The figure shows three views and two pictorial views of one solid part (mm, origin at its lowest corner). Answer the questions. Coordinates: 2 decimals unless noted, no trailing zeros. Order: outer loops, then holes, each group sorted by start corner. A loop starts at its lowest first (then second) coordinate and runs counter-clockwise, first axis right, second up.
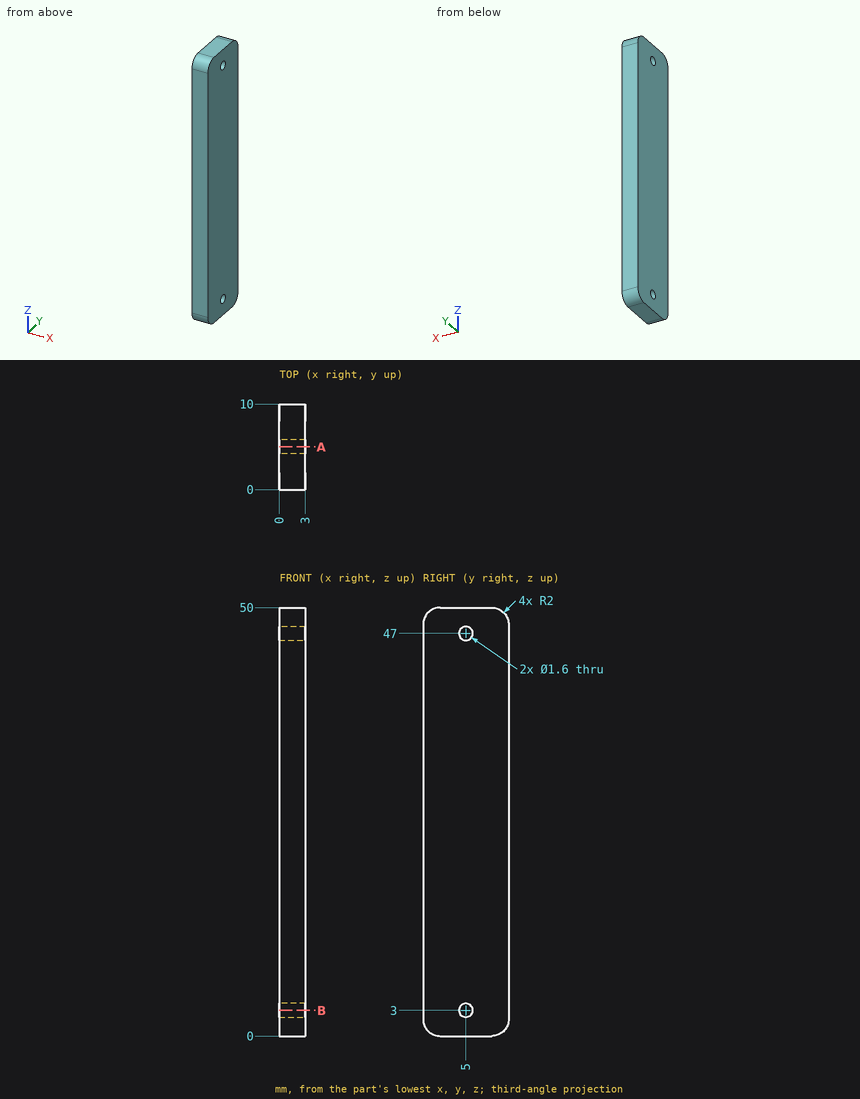
1) Straight lines are drawn through the part: probe 1 along Y at (x, z) = (1.75, 47); probe 2 along Z at (x, y) = (0.9, 1.75); probe 3 along Z at (x, y) = (2.25, 0.5). For each, find the intervals that lie inside material, in ascending order.
2) A cutting plane is placed at A-A, the plane y = 5. Write down the section's boundary in (x, z).
3) A cutting plane is placed at B-B, the plane z = 3. Write down the section's boundary in (x, y).
Working result:
1. probe 1: y = 0 to 4.2, 5.8 to 10
1. probe 2: z = 0.02 to 49.98
1. probe 3: z = 0.68 to 49.32
2. outline: (0, 0) - (3, 0) - (3, 2.2) - (0, 2.2) - close; (0, 3.8) - (3, 3.8) - (3, 46.2) - (0, 46.2) - close; (0, 47.8) - (3, 47.8) - (3, 50) - (0, 50) - close
3. outline: (0, 0) - (3, 0) - (3, 4.2) - (0, 4.2) - close; (0, 5.8) - (3, 5.8) - (3, 10) - (0, 10) - close
